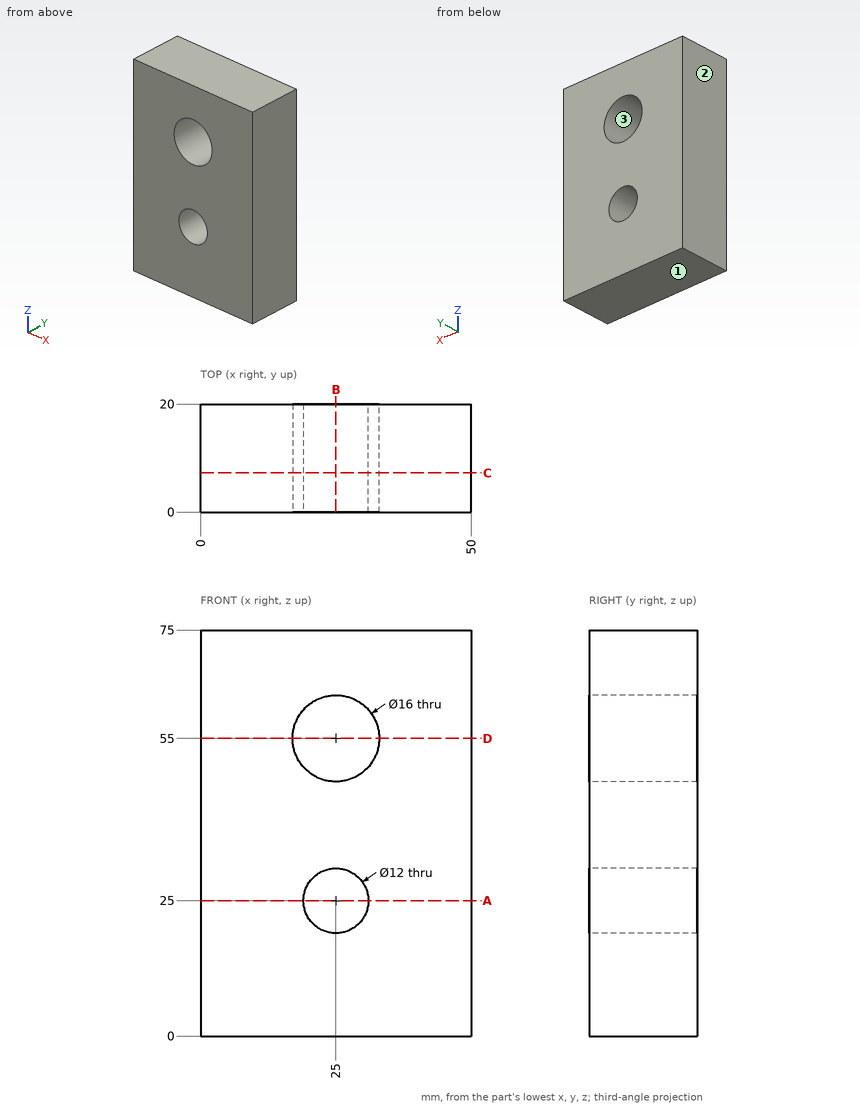
The drawing under review shows one solid part. Ordinate dimensions are in mm from its lowest x, y, z. Give positions to 0.01 mm unless a question says otherwise; leave off trailing zeros. Write each loop counter-clockwise with the first axis right and the second up, starting at its lowest first coordinate (ties: lowest second). Pieces come first, ordered by that corner, then holes.
1. For P1, Ø13, axis at x = 25, z = 55, coming from the +Y side, flat-tipped, find the tip position at first contact; note if it passes through.
2. Add section B-B, the plane x = 25. Write out the cut boundary in (y, z), plus the area to 3 significant figures.
3. Draft analysis for pull direction X (two halves, no side actions). For the marked faces 1, 2 and 3, state which applies: +X half, -X half, draft (parallel to the pull), parting line (faces both ways), or undercut.
4. Wall thickness on L1, parallel to Z at x = 25, y = 10.5; L2, parallel to X at y = 6.75, z = 25; L3, parallel to X at y = 10.75, z = 55: over which ranges is each line inside the solid? List them lowest first.
5. Add section A-A, the plane z = 25. Write out the cut boundary in (x, y).
6. Add section D-D, the plane z = 55. Write out the cut boundary in (x, y), plus the area to 3 significant figures.
7. Add section C-C, the plane y = 7.25. Write out the cut boundary in (x, z), plus the area to 3 significant figures.
Worked answers:
1. P1: passes through
2. outline: (0, 0) - (20, 0) - (20, 19) - (0, 19) - close; (0, 31) - (20, 31) - (20, 47) - (0, 47) - close; (0, 63) - (20, 63) - (20, 75) - (0, 75) - close
2. area: 940 mm2
3. face 1: draft
3. face 2: -X half
3. face 3: undercut
4. L1: z = 0 to 19, 31 to 47, 63 to 75
4. L2: x = 0 to 19, 31 to 50
4. L3: x = 0 to 17, 33 to 50
5. outline: (0, 0) - (19, 0) - (19, 20) - (0, 20) - close; (31, 0) - (50, 0) - (50, 20) - (31, 20) - close
6. outline: (0, 0) - (17, 0) - (17, 20) - (0, 20) - close; (33, 0) - (50, 0) - (50, 20) - (33, 20) - close
6. area: 680 mm2
7. outline: (0, 0) - (50, 0) - (50, 75) - (0, 75) - close; hole circle Ø16 at (25, 55); hole circle Ø12 at (25, 25)
7. area: 3,440 mm2
